Read the model definition and answer for the solid it produces. Units are mm, in the model's axes. A direction names the side the tool comes from. Round coordinates to 2 decimals unless told otherwise and drop trailing zeros. Write each loop counter-clockwise with the first axis right and the second up, starting at its lowest first coordinate (ties: lowest second). Pieces come first, ordered by that corner, then holes. Notation, with made-up numbers: (0, 15) - (35, 15) arc R19 cw to (35, 43) - close; hole circle Ø5 at (6, 81.5). An arc over 180 degrees is marked (long way). Answer as CSV lines item,"result". Start each with the question number.
1) Which of the six approach directions +Z, -Z, +X, -X, +Y, -Y give full straight-line access (tool end or side, diameter ignored) to faces 4 (the flat face through (182, -135, 381)), 5 (the flat face through (77.08, -76.41, 436.58)), 6 (the flat face through (-216, -112.5, 392))?
2) Find section C-C on x = -327.5. Determine the outline of the cut face in (y, z).
3) Find section A-A on z = 431. Determine the outline of the cut face in (x, y).
4) Each of these flat-tipped pins is pushed along its axis until it touches: pin 1 (5 mm diameter, centred on x = -217, z = 319, fed in from +Y); pin 2 (20 mm diameter, centred on x = -34, y = -95, fed in from +Z). Where does it stop, or does it pass through?
5) Find section B-B on y = -191.5. Determine the outline of the cut face in (x, z), then the cut area to 3 significant figures.
6) Find section D-D on z = 573.5. Determine the outline of the cut face in (x, y).
7) For a pull along Z with two mould halves and no side action, classify faces 1 (the flat face through (-385, 50, 719)), 2 (the flat face through (-480.17, -99.82, 469.91)), 3 (the flat face through (151, -99, 731.737)) as +Z half, -Z half, draft (parallel to the pull), parting line (faces both ways), or undercut.
8) Consider line 1 along Y through (x, z) = (237.5, 369); line 2 along Y through (x, z) = (-223.5, 651); line 3 along X through (y, z) = (-129, 209.5). Determine where each line is inside the solid, lowest interval first.
from build123d import *

# Parameters (mm, degrees)
F2_DEPTH      = 12.5
F3_DEPTH      = 35
F5_DEPTH      = 25
F6_DEPTH      = 12
F7_DEPTH      = 116
F7_DEPTH_BACK = 25
F8_DEPTH      = 25
F9_W          = 12
F9_H          = 137.5
F9_H_2        = 25
F10_DEPTH     = 25
F11_W         = 70
F11_H         = 33.2023501396
F12_DEPTH     = 25
F13_DEPTH     = 12.5
F14_W         = 25
F14_H         = 19.5178985596
F15_DEPTH     = 25
F16_R         = 56.3233112178
F16_R_2       = 12.5
F17_DEPTH     = 25
F19_R         = 58.1415954248
F20_DEPTH     = 25


with BuildPart() as f2:
    # F1 (on offset) → F2 (new body, symmetric)
    with BuildSketch(Plane.XZ.offset(100)):
        Polygon((-436.7461862998, 528.7278605353), (0, 184.4581483886), (152.0332864558, 681.7366214894), (-389.9667135442, 681.7366214894), align=None)
    extrude(amount=F2_DEPTH, both=True)

    # F1 (on offset) → F3 (join, symmetric)
    with BuildSketch(Plane.XZ.offset(100)):
        with BuildLine():
            Line((152.0332864558, 681.7366214894), (0, 184.4581483886))
            Line((0, 184.4581483886), (75.4155046728, 188.0290943346))
            ThreePointArc((75.4155046728, 188.0290943346), (118.345751191, 355.6091461552), (247.9658580263, 470.1722629873))
            Line((247.9658580263, 470.1722629873), (152.0332864558, 681.7366214894))
        make_face()
        with BuildLine():
            ThreePointArc((247.9658580263, 470.1722629873), (118.345751191, 355.6091461552), (75.4155046728, 188.0290943346))
            Line((75.4155046728, 188.0290943346), (369.5859169395, 201.9581483886))
            Line((369.5859169395, 201.9581483886), (247.9658580263, 470.1722629873))
        make_face()
    extrude(amount=F3_DEPTH, both=True)

    # F4 (on face) → F5 (join, symmetric)
    with BuildSketch(Plane.XY.offset(681.7366214894)):
        with BuildLine():
            Line((152.0332864558, -112.5), (152.0332864558, -87.5))
            ThreePointArc((152.0332864558, -87.5), (139.5332864558, -100), (152.0332864558, -112.5))
        make_face()
        with BuildLine():
            ThreePointArc((152.0332864558, -112.5), (160.8721212207, -108.8388347648), (164.5332864558, -100))
            ThreePointArc((164.5332864558, -100), (160.8721212207, -91.1611652352), (152.0332864558, -87.5))
            Line((152.0332864558, -87.5), (152.0332864558, -112.5))
        make_face()
    extrude(amount=F5_DEPTH, both=True)

    # F6 (add): a face of the model
    f6_faces = [f2.faces().sort_by_distance(p)[0] for p in [
        (-413.356449922, -100, 605.2322410124),
    ]]
    extrude(f6_faces, amount=F6_DEPTH)

    # F7 (add, two sides): a face of the model
    f7_faces = [f2.faces().sort_by_distance(p)[0] for p in [
        (-442.4840148356, -100, 530.4820907636),
    ]]
    extrude(f7_faces, amount=F7_DEPTH)
    extrude(f7_faces, amount=-F7_DEPTH_BACK)

    # F8 (add): a face of the model
    f8_faces = [f2.faces().sort_by_distance(p)[0] for p in [
        (-395.70454208, -100, 683.4908517177),
    ]]
    extrude(f8_faces, amount=F8_DEPTH)

    # F9 (on face) → F10 (join)
    with BuildSketch(Plane(origin=(164.5856050194, 0, 538.3352571426), x_dir=(0.956304756, 0, -0.2923717047), z_dir=(0.2923717047, 0, 0.956304756))):
        with Locations((-578.2475210263, -181.25)):
            Rectangle(F9_W, F9_H)
        with Locations((-578.2475210263, -18.75)):
            Rectangle(F9_W, F9_H)
        with Locations((-578.2475210263, -100)):
            Rectangle(F9_W, F9_H_2)
    extrude(amount=F10_DEPTH)

    # F11 (on face) → F12 (join)
    with BuildSketch(Plane(origin=(382.5134832971, 0, 173.4484124494), x_dir=(0, 1, 0), z_dir=(0.9107440224, 0, 0.4129713376))):
        with Locations((-100, 327.7641832829)):
            Rectangle(F11_W, F11_H)
    extrude(amount=F12_DEPTH)

    # F1 (on offset) → F13 (join, symmetric)
    with BuildSketch(Plane.XZ.offset(100)):
        with BuildLine():
            Line((-573.2489245515, 201.9581483886), (-278.8860573945, 192.9719122971))
            ThreePointArc((-278.8860573945, 192.9719122971), (-278.783209758, 197.4645072005), (-278.7489245515, 201.9581483886))
            ThreePointArc((-278.7489245515, 201.9581483886), (-328.1359004952, 365.2059827937), (-459.7326626701, 473.7012408279))
            Line((-459.7326626701, 473.7012408279), (-573.2489245515, 201.9581483886))
        make_face()
        with BuildLine():
            Line((-278.8860573945, 192.9719122971), (0, 184.4581483886))
            Line((0, 184.4581483886), (-436.7461862998, 528.7278605353))
            Line((-436.7461862998, 528.7278605353), (-459.7326626701, 473.7012408279))
            ThreePointArc((-459.7326626701, 473.7012408279), (-328.1359004952, 365.2059827937), (-278.7489245515, 201.9581483886))
            ThreePointArc((-278.7489245515, 201.9581483886), (-278.783209758, 197.4645072005), (-278.8860573945, 192.9719122971))
        make_face()
    extrude(amount=F13_DEPTH, both=True)

    # F14 (on face) → F15 (join)
    with BuildSketch(Plane(origin=(-558.7186830171, 0, 170.8174437025), x_dir=(0, -1, 0), z_dir=(-0.956304756, 0, 0.2923717047))):
        with Locations((100, 318.746984005)):
            Rectangle(F14_W, F14_H)
    extrude(amount=F15_DEPTH)

    # F19 (on face) → F20 (join)
    with BuildSketch(Plane.XY.offset(706.7366214894)):
        with Locations((152.0332864558, -100)):
            Circle(F19_R)
    extrude(amount=F20_DEPTH)


with BuildPart() as f17:
    # F16 (on face) → F17 (new body)
    with BuildSketch(Plane.XY.offset(706.7366214894)):
        with Locations((152.0332864558, -100)):
            Circle(F16_R)
        with Locations((152.0332864558, -100)):
            Circle(F16_R_2, mode=Mode.SUBTRACT)
    extrude(amount=F17_DEPTH)


solid = f2.part
Check values:
1,face 4,"-Z, +X, -X, -Y"
1,face 5,"-X, +Y"
1,face 6,"-X, -Y"
2,outline,"(-112.5, 194.46) - (-87.5, 194.46) - (-87.5, 681.74) - (-112.5, 681.74) - close"
3,outline,"(-479.17, -112.5) - (75.38, -112.5) - (75.38, -135) - (265.73, -135) - (265.73, -65) - (75.38, -65) - (75.38, -87.5) - (-479.17, -87.5) - close"
4,pin 1,"stops at y = -87.5"
4,pin 2,"stops at z = 681.74"
5,outline,"(-394.13, 709.15) - (-382.66, 705.64) - (-375.35, 729.55) - (-386.82, 733.06) - close"
5,area,"300 mm^2"
6,outline,"(-435.61, -112.5) - (118.94, -112.5) - (118.94, -135) - (201.11, -135) - (201.11, -65) - (118.94, -65) - (118.94, -87.5) - (-435.61, -87.5) - close"
7,face 1,"draft"
7,face 2,"undercut"
7,face 3,"+Z half"
8,line 1,"y = -135 to -65"
8,line 2,"y = -112.5 to -87.5"
8,line 3,"x = 7.66 to 366.17"
